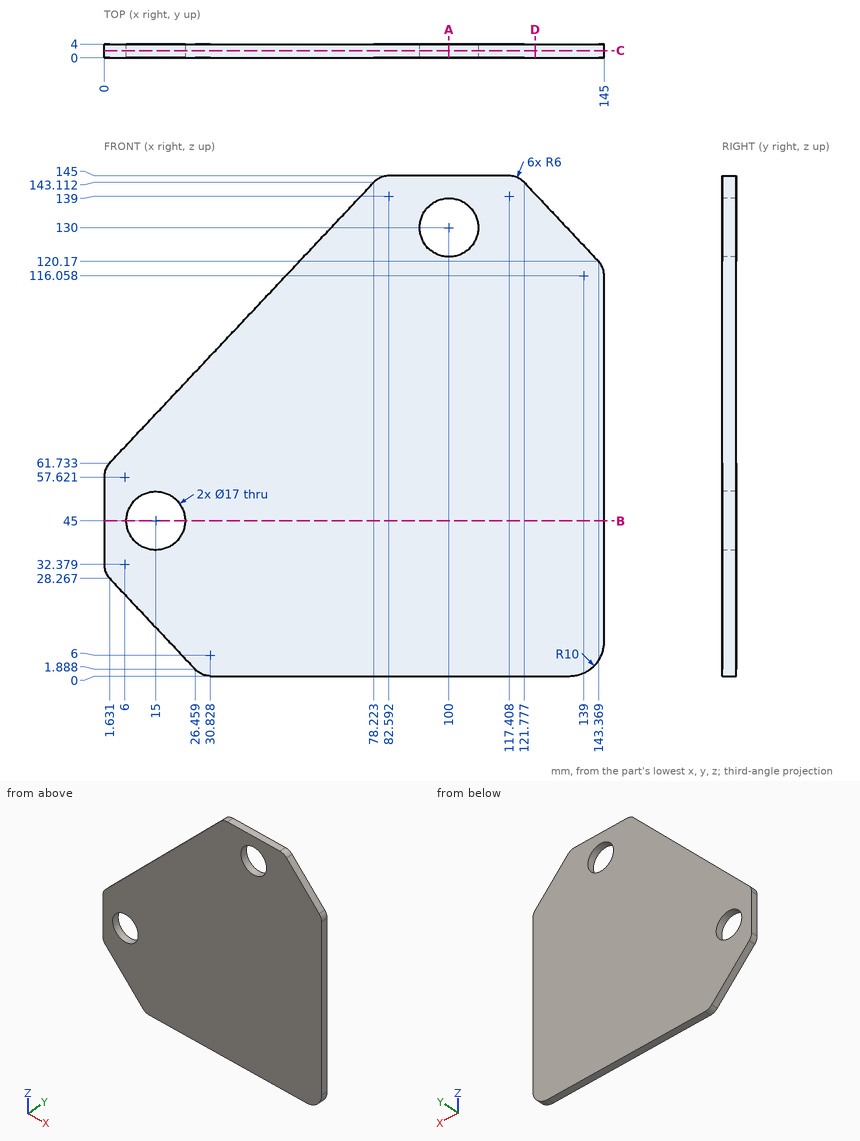
Drawing for the job (mm, zero at the part's lowest x, y, z). Give positions to 0.01 mm unless a question says otherwise; leave off trailing zeros. Order: outer loops, then holes, each group sorted by start corner. A loop starts at its lowest first (then second) coordinate and runs counter-clockwise, first axis right, second up. Notation, with made-up numbers: (32.5, -24) -> (61.5, -24) arc R30 cw to (61.5, 9) -> close; hole circle Ø8 at (70, 37). An arc over 180 degrees is marked (long way). Use one line per item in the form item = value.
(1) Saw through at A-A (x = 100). Write the cut outline in (y, z).
Solution:
outline = (0, 0) -> (4, 0) -> (4, 121.5) -> (0, 121.5) -> close; (0, 138.5) -> (4, 138.5) -> (4, 145) -> (0, 145) -> close
(2) Saw through at B-B (z = 45). Write the cut outline in (x, y).
Solution:
outline = (0, 0) -> (6.5, 0) -> (6.5, 4) -> (0, 4) -> close; (23.5, 0) -> (145, 0) -> (145, 4) -> (23.5, 4) -> close
(3) Drill centre lines: line 1 (Z direction, x = 100, y = 2.4); line 2 (Z direction, x = 15, y = 2.5) (1 decimal); line 3 (X direction, y = 2, z = 52.5). Where is each one in solid material? Low to high. Write a range as from..to.
Solution:
line_1 = 0..121.5, 138.5..145
line_2 = 14.1..36.5, 53.5..75.9
line_3 = 0..11, 19..145
(4) Flat gauge pins, fed straight in: P1, Ø2, axis at x = 116.5, z = 86, coming from the -Y side; P2, Ø15.5, axis at x = 15, z = 45, coming from the -Y side. Where does each tip first touch, or does it go through?
Solution:
P1 = 0
P2 = through
(5) Saw through at D-D (x = 125). Write the cut outline in (y, z).
Solution:
outline = (0, 0) -> (4, 0) -> (4, 139.69) -> (0, 139.69) -> close
(6) Saw through at C-C (y = 2.05). Write the cut outline in (x, z), then the cut area to 3 significant figures.
Solution:
outline = (0, 32.38) arc R6 ccw to (1.63, 28.27) -> (26.46, 1.89) arc R6 ccw to (30.83, 0) -> (135, 0) arc R10 ccw to (145, 10) -> (145, 116.06) arc R6 ccw to (143.37, 120.17) -> (121.78, 143.11) arc R6 ccw to (117.41, 145) -> (82.59, 145) arc R6 ccw to (78.22, 143.11) -> (1.63, 61.73) arc R6 ccw to (0, 57.62) -> close; hole circle Ø17 at (15, 45); hole circle Ø17 at (100, 130)
area = 16,400 mm²
